Build history of the part. All positions in model axes, mm. Round coordinates to 2 decimals unless told otherwise and drop trailing zeros. Loops run counter-clockwise (first coordinate to the right, second up) from the corner with the lowest first, then second, coordinate; pieces in that order, holes last. Notation, with made-up numbers: (7, -12) -> (36, -12) arc R21 ccw to (36, -7) -> close; hole circle Ø4 at (-2, -35). An arc over 180 degrees is marked (long way). Put each result on its own line as item: value. Start each with the question number.
Item 1: Drill centre lines: probe 1 along X at (y, z) = (-0.25, -10); probe 2 along Z at (x, y) = (116, -0.7); probe 3 along X at (y, z) = (-0.85, -113). Where is each one in solid material? Low to high. Write a range as [from, to].
Item 2: Cut at C-C, the plane y = -0.8. List the corners of the cut face in (x, z).
Item 3: Cut at B-B, the plane x = 116. List the corners of the cut face in (y, z).
Item 4: Cut at A-A, the plane z = -10. List the corners of the cut face in (x, y).
Item 5: Flat gauge pin, fed straight in: pin 1 Ø0.6 at (y, z) = (-1, 6.5) entering from +X. Where does the tip first touch, or does it go through?
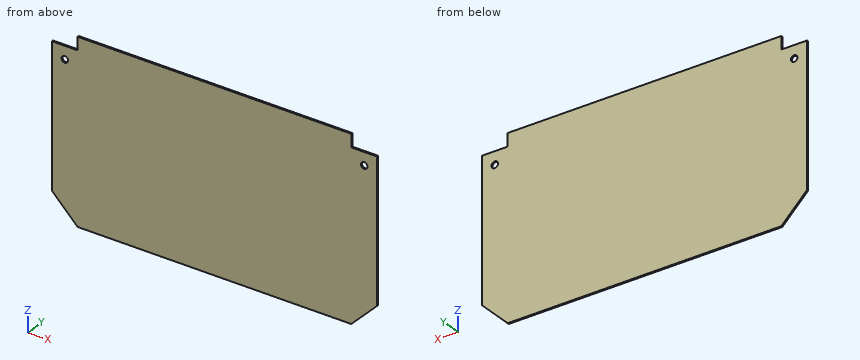
```python
from build123d import *

# Parameters (mm, degrees)
SKETCH_1_R             = 2.5
SM_BASE_FLANGE_1_DEPTH = 1.2


# Sheet-metal steps are written as plain solids
with BuildPart() as part:
    # Sketch 1 → 基材-凸緣1 (new body)
    with BuildSketch(Plane(origin=(0, 0, 0), x_dir=(1, 0, 0), z_dir=(0, 1, 0))):
        Polygon((-126, 0), (-106, 0), (-106, -10), (0, -10), (0, 130), (-106, 130), (-126, 110), align=None)
        with Locations(Location((-116, 10, 0), (0, 0, 270))):
            Circle(SKETCH_1_R, mode=Mode.SUBTRACT)
    extrude(amount=-SM_BASE_FLANGE_1_DEPTH)

    # 鏡射1: part across face


with BuildPart() as part_1:
    add(part.part)
    add(part.part.mirror(Plane(origin=(0, -0.6, -60), x_dir=(0, 0, 1), z_dir=(1, 0, 0))))


solid = part_1.part
```
Reply:
1. probe 1: x = [-126, -118.5], [-113.5, 113.5], [118.5, 126]
1. probe 2: z = [-120, -12.5], [-7.5, 0]
1. probe 3: x = [-123, 123]
2. outline: (-126, -110) -> (-106, -130) -> (106, -130) -> (126, -110) -> (126, 0) -> (106, 0) -> (106, 10) -> (-106, 10) -> (-106, 0) -> (-126, 0) -> close; hole circle Ø5 at (-116, -10); hole circle Ø5 at (116, -10)
3. outline: (-1.2, -120) -> (0, -120) -> (0, -12.5) -> (-1.2, -12.5) -> close; (-1.2, -7.5) -> (0, -7.5) -> (0, 0) -> (-1.2, 0) -> close
4. outline: (-126, -1.2) -> (-118.5, -1.2) -> (-118.5, 0) -> (-126, 0) -> close; (-113.5, -1.2) -> (113.5, -1.2) -> (113.5, 0) -> (-113.5, 0) -> close; (118.5, -1.2) -> (126, -1.2) -> (126, 0) -> (118.5, 0) -> close
5. pin 1: stops at x = 106
